Geometry: see drawing. Coordinates: mm, zero at the bounding-box minimum. A direction names the side the tool comes from. Give positions to 0.01 mm unless a question says otherwise; leave off trailing zeros. Order: outer loops, then holes, each group sorted by start corner. A loop starts at its lowest first (then second) coordinate and runs counter-clockwise, first axis right, second up. Notation, with made-up numbers: M 27.5,42.5 L 69.5,42.5 A20 ccw 69.5,74.5 Z; hole C -16,-40 d9. An arc over 180 degrees is marked long. Use a Markdown table: item, result.
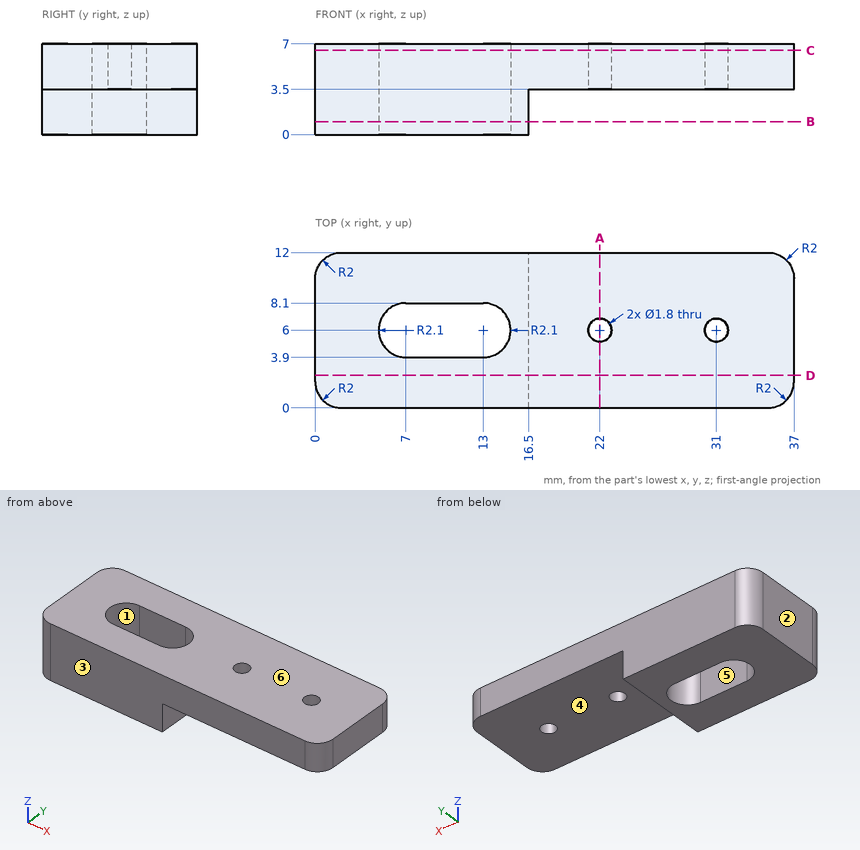
1) First-contact query: pin 1 Ø3 at (x, y) = (31, 6) entering from -Z; pin 2 Ø1 at (y, z) = (3, 1.5) entering from +X. Flat tips, straight axial feed; report the tip coordinate or a pass-through.
Response values:
| item | result |
|---|---|
| pin 1 | stops at z = 3.5 |
| pin 2 | stops at x = 16.5 |
2) Reachability of the marked faces 4, 5 and 6 from +Z, -Z, +X, -X, +Y, -Y: full face, straight path, thin tool, end or side. Return the list, or none.
Response values:
| item | result |
|---|---|
| face 4 | -Z, +X, +Y, -Y |
| face 5 | +Z, -Z |
| face 6 | +Z, +X, -X, +Y, -Y |
3) Cut plane A-A on x = 22. Return loops of the section in (y, z), and give its area (3 significant figures).
Response values:
| item | result |
|---|---|
| outline | M 0,3.5 L 5.1,3.5 L 5.1,7 L 0,7 Z; M 6.9,3.5 L 12,3.5 L 12,7 L 6.9,7 Z |
| area | 35.7 mm² |
4) Cut plane B-B on z = 1. Return loops of the section in (x, y).
Response values:
| item | result |
|---|---|
| outline | M 0,2 A2 ccw 2,0 L 16.5,0 L 16.5,12 L 2,12 A2 ccw 0,10 Z; hole M 7,3.9 L 13,3.9 A2.1 ccw 13,8.1 L 7,8.1 A2.1 ccw Z |
5) Material intervals for line 1 (X direction, y = 6, z = 5); line 2 (Y direction, x = 31, z = 6.35); line 3 (Y direction, x = 11, z = 4.5), sorted ascending. Write a range as from..to.
Response values:
| item | result |
|---|---|
| line 1 | x = 0..4.9, 15.1..21.1, 22.9..30.1, 31.9..37 |
| line 2 | y = 0..5.1, 6.9..12 |
| line 3 | y = 0..3.9, 8.1..12 |
6) Cut plane D-D on y = 2.5. Return loops of the section in (x, z).
Response values:
| item | result |
|---|---|
| outline | M 0,0 L 16.5,0 L 16.5,3.5 L 37,3.5 L 37,7 L 0,7 Z |
7) Mould query, pull axis Y, two halves, no side actions, for the marked faces 1, 2 and 3. Classes: released by +Y, released by -Y, zero draft, split by the parting line, or undercut.
Response values:
| item | result |
|---|---|
| face 1 | undercut |
| face 2 | zero draft |
| face 3 | released by -Y |
8) Cut plane C-C on z = 6.5. Return loops of the section in (x, y), and give its area (3 significant figures).
Response values:
| item | result |
|---|---|
| outline | M 0,2 A2 ccw 2,0 L 35,0 A2 ccw 37,2 L 37,10 A2 ccw 35,12 L 2,12 A2 ccw 0,10 Z; hole M 7,3.9 L 13,3.9 A2.1 ccw 13,8.1 L 7,8.1 A2.1 ccw Z; hole C 22,6 d1.8; hole C 31,6 d1.8 |
| area | 396 mm² |
